Could you check a few things on this model? Use its own coordinates, in mm. A direction names the side the tool comes from. Give positions to 0.01 mm unless a question says otherwise; leave off trailing zeros. Order: outer loops, then holes, each group sorted by start corner. A loop starts at its lowest first (then second) coordinate and runs counter-clockwise, first axis right, second up. Notation, with made-up numbers: M -2,-25 L 56,-25 A27 cw 56,-2 Z; hole C 65.25,12.25 d8. An arc over 180 degrees is marked long. Use a Markdown table: item, result. Add a question column.
Item 1: I'm going to push flat-ended pins straight in: pin 1 Ø1.8 at (y, z) = (17.78, 10.16) entering from -X; pin 2 Ø14 at (x, z) = (-15, -3.5) entering from +Y; pin 3 Ø8 at (y, z) = (18, -1) entering from -X; pin 4 Ø6 at (y, z) = (-5, -1) entering from +X. Where does each tip first touch, or does it pass through?
Item 2: Suppose I cut it at A-A on y = 5.08. Write out the boundary of the cut face in (x, z), plus the area to 3 significant figures.
Item 3: Suppose I cut it at D-D on y = 1. Write out the boundary of the cut face in (x, z).
Item 4: If we mould it in two halves opening along Y, with no side actions, what happens to faces 5 (the face through (-2.593, 16.766, 10.687)), 6 (the face through (-4, 2, 12.7)), 7 (the face through (0, 22.86, 0))? For each: released by +Y, released by -Y, zero draft, split by the parting line, or undercut.
Item 5: If I drill on L1, parallel to Z at x = -3, y = 5; L2, parallel to Y at x = -5.5, z = -10.5; L3, parallel to Y at x = -3, z = 10.16, over which ranges is the centre line in solid material (lowest first)? Write a range as from..to.
Item 6: For faces 1 (the face through (-6.35, 11, 0)), 2 (the face through (-6.528, -11.251, 11.172)), 3 (the face through (2.286, -8, -2)), 4 (the face through (1.27, 5, 10)), which set-ups out of +Z, -Z, +X, -X, +Y, -Y let a thin tool reach every point of the face, with its end or its side?
Item 7: Suppose I cut it at C-C on x = -11.25. Write out the boundary of the cut face in (y, z), plus the area to 3 significant figures.
Item 8: Suppose I cut it at B-B on z = -9.75. Write out the boundary of the cut face in (x, y).
from build123d import *

# Parameters (mm, degrees)
PROFILE_W               = 12.7
PROFILE_H               = 22.86
PROFILE_W_2             = 6.35
PROFILE_H_2             = 12.7
BOSS_EXTRUDE1_DEPTH     = 12.7
SKETCH7_W               = 19.05
SKETCH7_H               = 12.7
BOSS_EXTRUDE2_DEPTH     = 25.4
SCREWHOLE_R             = 2.159
CUT_EXTRUDE1_DEPTH      = 1
CUT_EXTRUDE1_DEPTH_BACK = 26.4
SKETCH3_R               = 3.683
SKETCH3_R_2             = 2.159
CUT_EXTRUDE2_DEPTH      = 4.064
SKETCH10_R              = 1.143
CUT_EXTRUDE3_DEPTH      = 7.62
FILLET6_R               = 5.08


with BuildPart() as part:
    # Profile → Boss-Extrude1 (new body, symmetric)
    with BuildSketch(Plane.XY):
        with Locations((0, 11.43)):
            Rectangle(PROFILE_W, PROFILE_H)
        with Locations((3.175, -6.35)):
            Rectangle(PROFILE_W_2, PROFILE_H_2)
    extrude(amount=BOSS_EXTRUDE1_DEPTH, both=True)

    # Sketch7 → Boss-Extrude2 (add)
    with BuildSketch(Plane.XY.offset(12.7)):
        with Locations((-9.525, -6.35)):
            Rectangle(SKETCH7_W, SKETCH7_H)
    extrude(amount=-BOSS_EXTRUDE2_DEPTH)

    # ScrewHole → Cut-Extrude1 (cut, two sides)
    with BuildSketch(Plane.ZY.offset(19.05)) as cut_extrude1_sk:
        with Locations((0, -6.477)):
            Circle(SCREWHOLE_R)
    extrude(amount=CUT_EXTRUDE1_DEPTH, mode=Mode.SUBTRACT)
    extrude(cut_extrude1_sk.sketch, amount=-CUT_EXTRUDE1_DEPTH_BACK, mode=Mode.SUBTRACT)

    # Sketch3 → Cut-Extrude2 (cut)
    with BuildSketch(Plane(origin=(6.35, 0, 0), x_dir=(0, 0, -1), z_dir=(1, 0, 0))):
        with Locations((0, -6.477)):
            Circle(SKETCH3_R)
        with Locations((0, -6.477)):
            Circle(SKETCH3_R_2, mode=Mode.SUBTRACT)
    extrude(amount=-CUT_EXTRUDE2_DEPTH, mode=Mode.SUBTRACT)

    # Sketch10 → Cut-Extrude3 (cut)
    with BuildSketch(Plane.ZY.offset(6.35)):
        with Locations((-10.16, 17.78)):
            Circle(SKETCH10_R)
        with Locations((10.16, 17.78)):
            Circle(SKETCH10_R)
        with Locations((10.16, 5.08)):
            Circle(SKETCH10_R)
        with Locations((-10.16, 5.08)):
            Circle(SKETCH10_R)
    extrude(amount=-CUT_EXTRUDE3_DEPTH, mode=Mode.SUBTRACT)

    # Fillet6
    fillet6_edges = [part.edges().sort_by_distance(p)[0] for p in [
        (0, 22.86, -12.7),
        (0, 22.86, 12.7),
        (-6.35, -12.7, 12.7),
        (-6.35, -12.7, -12.7),
    ]]
    fillet(fillet6_edges, radius=FILLET6_R)


solid = part.part
Findings below:
| question | item | result |
|---|---|---|
| 1 | pin 1 | stops at x = 1.27 |
| 1 | pin 2 | stops at y = 0 |
| 1 | pin 3 | stops at x = -6.35 |
| 1 | pin 4 | stops at x = 6.35 |
| 2 | outline | M -6.35,-12.7 L 6.35,-12.7 L 6.35,12.7 L -6.35,12.7 L -6.35,11.3 L 1.27,11.3 L 1.27,9.02 L -6.35,9.02 L -6.35,-9.02 L 1.27,-9.02 L 1.27,-11.3 L -6.35,-11.3 Z |
| 2 | area | 288 mm^2 |
| 3 | outline | M -6.35,-12.7 L 6.35,-12.7 L 6.35,12.7 L -6.35,12.7 Z |
| 4 | face 5 | undercut |
| 4 | face 6 | zero draft |
| 4 | face 7 | released by +Y |
| 5 | L1 | z = -12.7..-11.3, -9.02..9.02, 11.3..12.7 |
| 5 | L2 | y = -11.8..3.99, 6.17..16.69, 18.87..21.96 |
| 5 | L3 | y = -12.02..3.94, 6.22..16.64, 18.92..22.18 |
| 6 | face 1 | +Z, -Z, -X, +Y |
| 6 | face 2 | +Z, +X, -X, -Y |
| 6 | face 3 | +X |
| 6 | face 4 | -X |
| 7 | outline | M -12.7,-7.62 A5.08 ccw -7.62,-12.7 L 0,-12.7 L 0,12.7 L -7.62,12.7 A5.08 ccw -12.7,7.62 Z; hole C -6.48,0 d4.32 |
| 7 | area | 297 mm^2 |
| 8 | outline | M -19.05,-12.23 L 6.35,-12.23 L 6.35,22.39 L -6.35,22.39 L -6.35,18.85 L 1.27,18.85 L 1.27,16.71 L -6.35,16.71 L -6.35,6.15 L 1.27,6.15 L 1.27,4.01 L -6.35,4.01 L -6.35,0 L -19.05,0 Z |
